from build123d import *

# Parameters (mm, degrees)
SKETCH1_W           = 40
SKETCH1_H           = 40
SKETCH1_R           = 1.6
BOSS_EXTRUDE1_DEPTH = 1.5
SKETCH3_W           = 40
SKETCH3_H           = 1.5
BOSS_EXTRUDE2_DEPTH = 45.5
CUT_EXTRUDE1_DEPTH  = 64.798510954
SKETCH5_R           = 7
CUT_EXTRUDE2_DEPTH  = 64.798510954


with BuildPart() as part:
    # Sketch1 → Boss-Extrude1 (new body)
    with BuildSketch(Plane.XY):
        Rectangle(SKETCH1_W, SKETCH1_H)
        with Locations((14.9, 13.5)):
            Circle(SKETCH1_R, mode=Mode.SUBTRACT)
        with Locations(Location((-14.9, 13.5, 0), (0, 0, 180))):
            Circle(SKETCH1_R, mode=Mode.SUBTRACT)
        with Locations((15.1, -10.399163165)):
            Circle(SKETCH1_R, mode=Mode.SUBTRACT)
        with Locations(Location((-15.1, -10.399163165, 0), (0, 0, 180))):
            Circle(SKETCH1_R, mode=Mode.SUBTRACT)
    extrude(amount=BOSS_EXTRUDE1_DEPTH)

    # Sketch3 → Boss-Extrude2 (add)
    with BuildSketch(Plane(origin=(0, 0, 0), x_dir=(-1, 0, 0), z_dir=(0, 0, -1))):
        with Locations((0, 19.25)):
            Rectangle(SKETCH3_W, SKETCH3_H)
    extrude(amount=BOSS_EXTRUDE2_DEPTH)

    # Sketch4 → Cut-Extrude1 (cut, through all)
    with BuildSketch(Plane(origin=(0, 20, 0), x_dir=(1, 0, 0), z_dir=(0, 1, 0))):
        with BuildLine():
            ThreePointArc((0, 45.5), (14.142135624, 39.642135624), (20, 25.5))
            Line((20, 25.5), (20, 45.5))
            Line((20, 45.5), (0, 45.5))
        make_face()
        with BuildLine():
            Line((-20, 45.5), (-20, 25.5))
            ThreePointArc((-20, 25.5), (-14.142135624, 39.642135624), (0, 45.5))
            Line((0, 45.5), (-20, 45.5))
        make_face()
    extrude(amount=-CUT_EXTRUDE1_DEPTH, mode=Mode.SUBTRACT)

    # Sketch5 → Cut-Extrude2 (cut, through all)
    with BuildSketch(Plane(origin=(0, 20, 0), x_dir=(1, 0, 0), z_dir=(0, 1, 0))):
        with Locations(Location((0, 19, 0), (0, 0, 270))):
            Circle(SKETCH5_R)
    extrude(amount=-CUT_EXTRUDE2_DEPTH, mode=Mode.SUBTRACT)


solid = part.part
Check sheet for the modelled part. Datum: model origin and axes. Units: mm. A direction names the side the tool comes from. Give positions to 0.01 mm unless a question says otherwise; leave off trailing zeros. Write each loop counter-clockwise with the first axis right and the second up, starting at its lowest first coordinate (ties: lowest second). Pieces come first, ordered by that corner, then holes. Notation, with made-up numbers: (86.5, 41.25) -> (138.5, 41.25) arc R21 cw to (138.5, 60.25) -> close; hole circle Ø10 at (-15.75, 60). An arc over 180 degrees is marked (long way). One line per item, written item: value. Start each with the question number.
Item 1: Section check C-C on y = 14.5. Record the cut outline in (x, z).
Item 2: Gauge pin test, flat ends, axial feed: pin 1 (5 mm diameter, centred on x = -15.1, y = -10.4, fed in from +Z); pin 2 (4 mm diameter, centred on x = -4, z = -29.5, fed in from -Y); pin 3 (12 mm diameter, centred on x = 5.5, y = -8.5, fed in from -Z). Record the tip position at first contact, or that the pin passes through.
Item 3: Draft check along X on faces 3 (the cylindrical face through (16.426, 13.981, 0.74)), 4 (the cylindrical face through (0, 19, -26)), 5 (the flat face through (-20, 6, 1)), 6 (the flat face through (0, -20, 1)). Enter one of: +X half, -X half, draft (parallel to the pull), parting line (faces both ways), or undercut.
Item 4: Section check A-A on z = -19. Record the cut outline in (x, y).
Item 5: Section check B-B on x = -14.9. Record the cut outline in (y, z).
Item 6: Tool access check on faces 1 (the flat face through (0, 0, 0)), 2 (the cylindrical face through (16.58, -11.01, 0.74)). Record the directions out of +Z, -Z, +X, -X, +Y, -Y that give a thin tool (end or side, any length) a straight path to the whole face; none if there is none.
Item 7: Section check D-D on x = -6. Record the cut outline in (y, z), then the cut area to 3 significant figures.
Item 8: Material ranges on probe 1 along Y at (x, z) = (-14, 1); probe 2 along Z at (x, y) = (-13, 10.5); probe 3 along Y at (x, z) = (-3, -10), recorded low to high. Write a range as from..to.
Results list:
1. outline: (-20, 0) -> (-16.15, 0) -> (-16.15, 1.5) -> (-20, 1.5) -> close; (-13.65, 0) -> (13.65, 0) -> (13.65, 1.5) -> (-13.65, 1.5) -> close; (16.15, 0) -> (20, 0) -> (20, 1.5) -> (16.15, 1.5) -> close
2. pin 1: z = 1.5
2. pin 2: y = 18.5
2. pin 3: z = 0
3. face 3: undercut
3. face 4: undercut
3. face 5: -X half
3. face 6: draft
4. outline: (-20, 18.5) -> (-7, 18.5) -> (-7, 20) -> (-20, 20) -> close; (7, 18.5) -> (20, 18.5) -> (20, 20) -> (7, 20) -> close
5. outline: (-20, 0) -> (-11.99, 0) -> (-11.99, 1.5) -> (-20, 1.5) -> close; (-8.81, 0) -> (11.9, 0) -> (11.9, 1.5) -> (-8.81, 1.5) -> close; (15.1, 0) -> (18.5, 0) -> (18.5, -38.84) -> (20, -38.84) -> (20, 1.5) -> (15.1, 1.5) -> close
6. face 1: -Z, +X, -X, -Y
6. face 2: +Z, -Z
7. outline: (-20, 0) -> (18.5, 0) -> (18.5, -15.39) -> (20, -15.39) -> (20, 1.5) -> (-20, 1.5) -> close; (18.5, -44.58) -> (20, -44.58) -> (20, -22.61) -> (18.5, -22.61) -> close
7. area: 116 mm²
8. probe 1: -20..-11.56, -9.24..12.18, 14.82..20
8. probe 2: 0..1.5
8. probe 3: 18.5..20
